Build history of the part. All positions in model axes, mm. Give positions to 0.01 mm unless a question says otherwise; leave off trailing zeros. Order: outer loops, then holes, each group sorted by start corner. A loop starts at its lowest first (then second) coordinate and runs counter-clockwise, first axis right, second up. Notation, with made-up numbers: M 50,78 L 81,78 A22 cw 81,91 Z; hole C 41,-12.75 d7. An arc over 180 degrees is marked long. Answer as CSV lines item,"result".
from build123d import *

# Parameters (mm, degrees)
F1_DEPTH = 18
F5_DEPTH = 18
F7_DEPTH = 18


with BuildPart() as f1:
    # F0 (on Front) → F1 (new body)
    with BuildSketch(Plane.XZ):
        with BuildLine():
            Line((0, 675), (0, 0))
            Line((0, 0), (100, 0))
            Line((100, 0), (100, 275))
            ThreePointArc((100, 275), (114.644661, 310.355339), (150, 325))
            Line((150, 325), (650, 325))
            ThreePointArc((650, 325), (685.355339, 310.355339), (700, 275))
            Line((700, 275), (700, 0))
            Line((700, 0), (800, 0))
            Line((800, 0), (800, 850))
            Line((800, 850), (500, 1000))
            Line((500, 1000), (0, 675))
        make_face()
        with BuildLine():
            Line((650, 385), (150, 385))
            ThreePointArc((150, 385), (114.644661, 399.644661), (100, 435))
            Line((100, 435), (100, 535))
            Line((100, 535), (700, 535))
            Line((700, 535), (700, 435))
            ThreePointArc((700, 435), (685.355339, 399.644661), (650, 385))
        make_face(mode=Mode.SUBTRACT)
    extrude(amount=F1_DEPTH)

    # F4 (on face) → F5 (cut, through all)
    with BuildSketch(Plane.XZ.offset(18)):
        Polygon((458.077819, 972.750582), (416.155638, 945.501165), (425.965429, 930.40918), (467.887609, 957.658597), align=None)
    extrude(amount=-F5_DEPTH, mode=Mode.SUBTRACT)

    # F6 (on face) → F7 (cut, through all)
    with BuildSketch(Plane.XZ.offset(18)):
        Polygon((857.770876, 821.114562), (500, 1000), (491.950155, 983.900311), (849.721032, 805.014872), align=None)
    extrude(amount=-F7_DEPTH, mode=Mode.SUBTRACT)


solid = f1.part
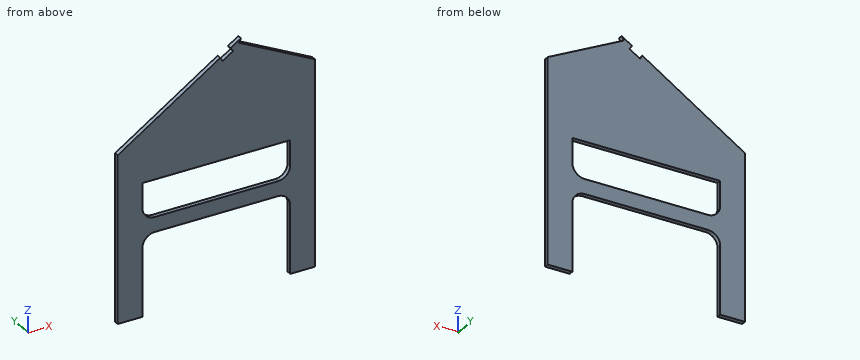
Item 1: Band-saw the part on B-B (z = 458). Give the cut face in (x, y).
Geometry says:
outline,"M 0,-18 L 100,-18 L 100,0 L 0,0 Z; M 700,-18 L 800,-18 L 800,0 L 700,0 Z"
Item 2: Band-saw the part on C-C (y = -5.5). Give the cut face in (x, z).
Geometry says:
outline,"M 0,0 L 100,0 L 100,275 A50 cw 150,325 L 650,325 A50 cw 700,275 L 700,0 L 800,0 L 800,829.88 L 491.95,983.9 L 425.97,930.41 L 416.16,945.5 L 0,675 Z; hole M 100,435 A50 ccw 150,385 L 650,385 A50 ccw 700,435 L 700,535 L 100,535 Z"
Item 3: Band-saw the part on D-D (x = 62.5). Give the cut face in (y, z) (3 decimals), and give its area (3 significant figures).
Geometry says:
outline,"M -18,0 L 0,0 L 0,715.625 L -18,715.625 Z"
area,"12,900 mm2"
Item 4: Drop flat-ended pins along their axis: pin 1 (6 mm diameter, centred on x = 219.5, y = -15, fed in from -Z); pin 2 (5 mm diameter, centred on y = -16, z = 868.5, fed in from -X); pin 3 (6 mm diameter, centred on y = -15, z = 701, fed in from -X). Give the stop position or say it passes through.
Geometry says:
pin 1,"stops at z = 325"
pin 2,"stops at x = 293.85"
pin 3,"stops at x = 35.38"
Item 5: Probe line 1 along X through (y, z) = (-2.25, 494); line 2 along Z through (x, y) = (231, -1.5); line 3 along Z through (x, y) = (164.5, -10.25) (3 decimals). List the from-to ranges inside material, lowest first. Write a range as from..to.
Geometry says:
line 1,"x = 0..100, 700..800"
line 2,"z = 325..385, 535..825.15"
line 3,"z = 325..385, 535..781.925"
Item 6: Band-saw the part on A-A (x = 357). Give the cut face in (y, z), and give its area (3 significant figures).
Geometry says:
outline,"M -18,325 L 0,325 L 0,385 L -18,385 Z; M -18,535 L 0,535 L 0,907.05 L -18,907.05 Z"
area,"7,780 mm2"
